Study the drawing (mm; zero at the part's minimum x, y, z) and answer. Coordinates: 2 decimals unless noted, no trailing zeros. Write each loop counter-clockwise with the first axis right and the second up, starting at its lowest first coordinate (ties: lowest second). Pieces come first, ordered by that corner, then holes. Notation, with made-up numbers: (64.25, 1) -> (123.25, 1) arc R14 ccw to (123.25, 23) -> close; hole circle Ø5 at (2.25, 26.25). An arc over 180 degrees is marked (long way). Write item = value, one per line. Start each with the question number.
1) Section D-D (x = 12) is taken. Count the separate pieces of the cut face and the enclosed holes in it, plus the area to 3 significant figures.
2) Section B-B (x = 8.5) is taken. Determine the outline of the cut face in (y, z).
3) Section C-C (z = 30) is taken. Determine the outline of the cut face in (x, y), plus the area to 3 significant figures.
4) For a pull along Y with two mould halves and no side action, classify the marked faces 1, 2, 3 and 4 as released by +Y, released by -Y, zero draft, split by the parting line, or undercut.
5) Flat-ended cylindrical pins translate along their axes: pin 1 Ø2.5 at (x, z) = (12, 37) entering from +Y; pin 2 Ø4.5 at (y, z) = (7.5, 23) entering from +X. Find the tip coordinate at first contact, or state that the pin passes through.
6) Section A-A (z = 17) is taken. Determine the outline of the cut face in (x, y), plus the area to 3 significant figures.
7) Find the intervals of material crossed by line 1 along Z through (x, y) = (12, 3.8); line 2 along Y through (x, z) = (13.5, 10); line 3 along X through (y, z) = (11.6, 17), in increasing order. Write a range as from..to.
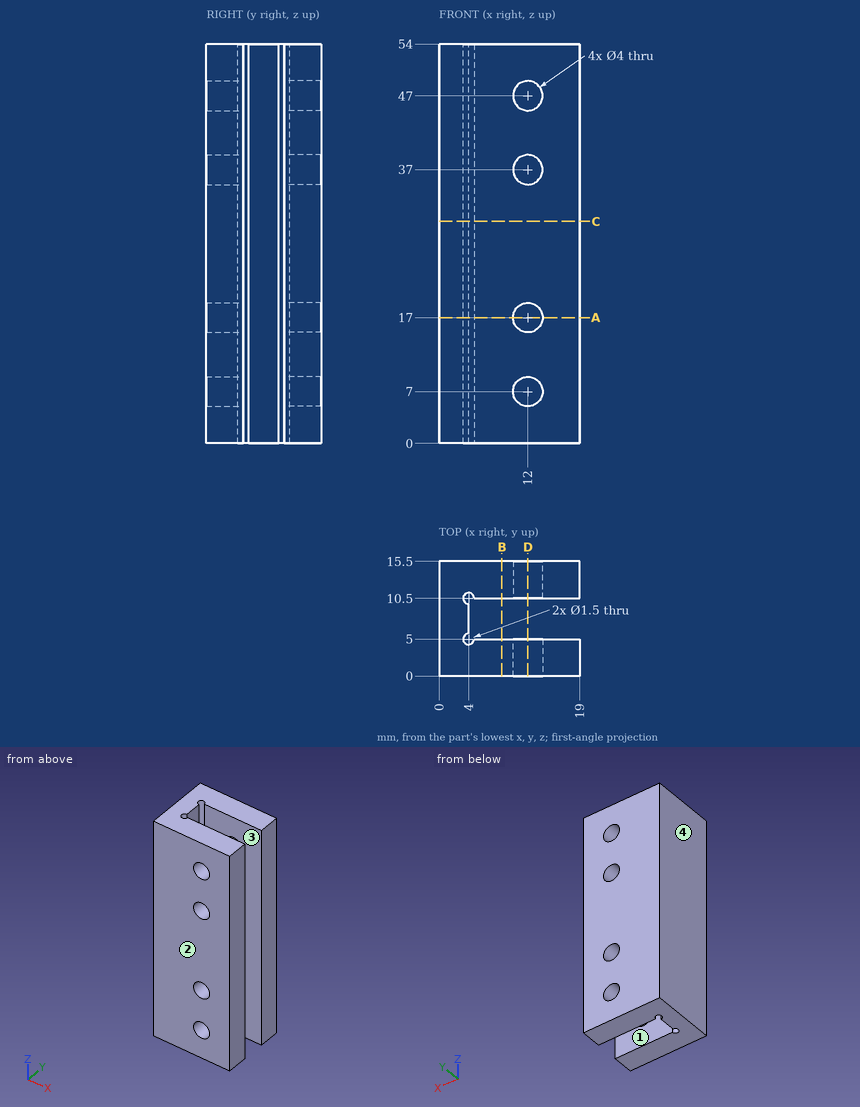
Answer key:
q1.separate_pieces = 10
q1.enclosed_holes = 0
q1.area = 380 mm^2
q2.outline = (0, 0) -> (5, 0) -> (5, 54) -> (0, 54) -> close; (10.5, 0) -> (15.5, 0) -> (15.5, 54) -> (10.5, 54) -> close
q3.outline = (0, 0) -> (19, 0) -> (19, 5) -> (4.75, 5) arc R0.75 cw (long way) to (4, 5.75) -> (4, 9.75) arc R0.75 cw (long way) to (4.75, 10.5) -> (19, 10.5) -> (19, 15.5) -> (0, 15.5) -> close
q3.area = 209 mm^2
q4.face_1 = undercut
q4.face_2 = released by -Y
q4.face_3 = undercut
q4.face_4 = zero draft
q5.pin_1 = through
q5.pin_2 = 4
q6.outline = (0, 0) -> (10, 0) -> (10, 5) -> (4.75, 5) arc R0.75 cw (long way) to (4, 5.75) -> (4, 9.75) arc R0.75 cw (long way) to (4.75, 10.5) -> (10, 10.5) -> (10, 15.5) -> (0, 15.5) -> close; (14, 0) -> (19, 0) -> (19, 5) -> (14, 5) -> close; (14, 10.5) -> (19, 10.5) -> (19, 15.5) -> (14, 15.5) -> close
q6.area = 169 mm^2
q7.line_1 = 0..5, 9..15, 19..35, 39..45, 49..54
q7.line_2 = 0..5, 10.5..15.5
q7.line_3 = 0..10, 14..19
